Input: part model. Units: mm. Frame: model coordinates. Face numbers are marked on the shaded views. A direction names the side the tool comes from. Round coordinates to 2 decimals unless told otherwise and drop trailing zeros. Order: outer loops, then holes, each group sorted by start corner. A loop starts at its lowest first (then second) coordinate and runs counter-clockwise, first axis right, second up. Notation, with made-up numbers: (57, 66.25) - (107, 66.25) arc R14 cw to (107, 86.25) - close; hole circle Ø11 at (67, 54.5). An arc over 180 degrees is marked (long way). One line per item, written item: value. Start each with the question number.
from build123d import *

# Parameters (mm, degrees)
SKETCH1_R           = 3.4
BOSS_EXTRUDE1_DEPTH = 40


with BuildPart() as part:
    # Sketch1 → Boss-Extrude1 (new body)
    with BuildSketch(Plane(origin=(0, 0, 0), x_dir=(1, 0, 0), z_dir=(0, 1, 0))):
        with BuildLine():
            Line((5.8, 4.385786438), (5.8, -4.385786438))
            Line((5.8, -4.385786438), (9.664213562, -8.25))
            Line((9.664213562, -8.25), (12.8, -8.25))
            Line((12.8, -8.25), (12.8, -4.1))
            Line((12.8, -4.1), (15, -4.1))
            Line((15, -4.1), (15, -12.5))
            ThreePointArc((15, -12.5), (14.267766953, -14.267766953), (12.5, -15))
            Line((12.5, -15), (4.1, -15))
            Line((4.1, -15), (4.1, -12.8))
            Line((4.1, -12.8), (8.25, -12.8))
            Line((8.25, -12.8), (8.25, -9.664213562))
            Line((8.25, -9.664213562), (4.385786438, -5.8))
            Line((4.385786438, -5.8), (-4.385786438, -5.8))
            Line((-4.385786438, -5.8), (-8.25, -9.664213562))
            Line((-8.25, -9.664213562), (-8.25, -12.8))
            Line((-8.25, -12.8), (-4.1, -12.8))
            Line((-4.1, -12.8), (-4.1, -15))
            Line((-4.1, -15), (-12.5, -15))
            ThreePointArc((-12.5, -15), (-14.267766953, -14.267766953), (-15, -12.5))
            Line((-15, -12.5), (-15, -4.1))
            Line((-15, -4.1), (-12.8, -4.1))
            Line((-12.8, -4.1), (-12.8, -8.25))
            Line((-12.8, -8.25), (-9.664213562, -8.25))
            Line((-9.664213562, -8.25), (-5.8, -4.385786438))
            Line((-5.8, -4.385786438), (-5.8, 4.385786438))
            Line((-5.8, 4.385786438), (-9.664213562, 8.25))
            Line((-9.664213562, 8.25), (-12.8, 8.25))
            Line((-12.8, 8.25), (-12.8, 4.1))
            Line((-12.8, 4.1), (-15, 4.1))
            Line((-15, 4.1), (-15, 12.5))
            ThreePointArc((-15, 12.5), (-14.267766953, 14.267766953), (-12.5, 15))
            Line((-12.5, 15), (-4.1, 15))
            Line((-4.1, 15), (-4.1, 12.8))
            Line((-4.1, 12.8), (-8.25, 12.8))
            Line((-8.25, 12.8), (-8.25, 9.664213562))
            Line((-8.25, 9.664213562), (-4.385786438, 5.8))
            Line((-4.385786438, 5.8), (4.385786438, 5.8))
            Line((4.385786438, 5.8), (8.25, 9.664213562))
            Line((8.25, 9.664213562), (8.25, 12.8))
            Line((8.25, 12.8), (4.1, 12.8))
            Line((4.1, 12.8), (4.1, 15))
            Line((4.1, 15), (12.5, 15))
            ThreePointArc((12.5, 15), (14.267766953, 14.267766953), (15, 12.5))
            Line((15, 12.5), (15, 4.1))
            Line((15, 4.1), (12.8, 4.1))
            Line((12.8, 4.1), (12.8, 8.25))
            Line((12.8, 8.25), (9.664213562, 8.25))
            Line((9.664213562, 8.25), (5.8, 4.385786438))
        make_face()
        Circle(SKETCH1_R, mode=Mode.SUBTRACT)
    extrude(amount=BOSS_EXTRUDE1_DEPTH)


solid = part.part
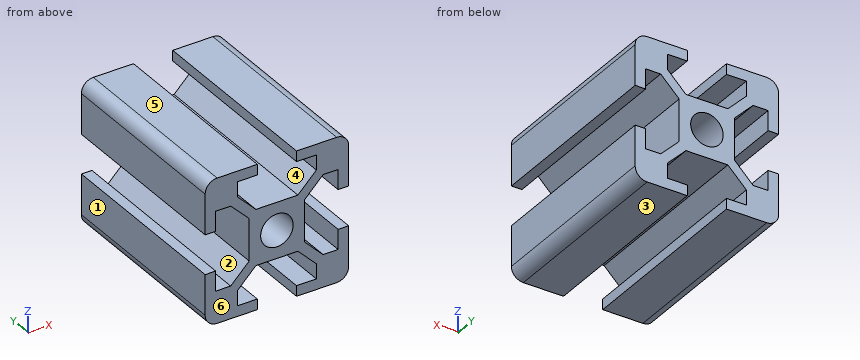
Item 1: Pull-direction query (Z, two-part tool) for the marked faces 3, 4, 5 and 6; classes: released by +Z, released by -Z, zero draft, split by the parting line, or undercut.
Item 2: Section query C-C on x = -7. Return loops of the section in (y, z).
Item 3: Section query B-B on x = 0. Return loops of the section in (y, z), and give its area (3 significant figures).
Item 4: Line query: L1, parallel to X at y = 15, z = 0; L2, parallel to Z at x = 8, y = 35.5. Output: solid intervals per line, ascending.
Item 5: Reachability of the marked faces 1 and 2 from +Z, -Z, +X, -X, +Y, -Y: full face, straight path, thin tool, end or side. Return the list, or none.
Item 6: First-contact query: pin 1 Ø10 at (x, y) = (-4, 14) entering from +Z; pin 2 Ø4.5 at (y, z) = (29, -1) entering from -X; pin 3 Ø1.8 at (x, y) = (-14, 22.5) entering from -Z; pin 4 Ø1.8 at (y, z) = (28, -14) entering from +X. Flat tips, straight axial feed; report the tip coordinate or a pass-through.
Item 7: Section query A-A on z = 0. Return loops of the section in (x, y).
Geometry results:
1. face 3: released by -Z
1. face 4: undercut
1. face 5: released by +Z
1. face 6: zero draft
2. outline: (0, -15) - (40, -15) - (40, -12.8) - (0, -12.8) - close; (0, -8.41) - (40, -8.41) - (40, -5.59) - (0, -5.59) - close; (0, 5.59) - (40, 5.59) - (40, 8.41) - (0, 8.41) - close; (0, 12.8) - (40, 12.8) - (40, 15) - (0, 15) - close
3. outline: (0, -5.8) - (40, -5.8) - (40, -3.4) - (0, -3.4) - close; (0, 3.4) - (40, 3.4) - (40, 5.8) - (0, 5.8) - close
3. area: 192 mm^2
4. L1: x = -5.8 to -3.4, 3.4 to 5.8
4. L2: z = -15 to -12.8, -9.41 to -6.59, 6.59 to 9.41, 12.8 to 15
5. face 1: +Z, -Z, -X, +Y, -Y
5. face 2: +Y, -Y
6. pin 1: stops at z = 15
6. pin 2: stops at x = -5.8
6. pin 3: stops at z = -14.93
6. pin 4: stops at x = 14.93
7. outline: (-5.8, 0) - (-3.4, 0) - (-3.4, 40) - (-5.8, 40) - close; (3.4, 0) - (5.8, 0) - (5.8, 40) - (3.4, 40) - close
